Read the model definition and answer for the solid it produces. Units are mm, in the model's axes. Coordinates: 2 decimals unless noted, no trailing zeros. Write each loop counter-clockwise with the first axis right and the second up, starting at its lowest first coordinate (ties: lowest second). Pieces come first, ordered by that corner, then holes. Notation, with made-up numbers: (39.25, 61) -> (62.25, 61) arc R10 ccw to (62.25, 77) -> close; hole circle Ø10 at (62.25, 65.5). An arc over 180 degrees is marked (long way). Answer in a Markdown table with one row per item. Add a question column.
Item 1: Straight lines are drawn through the part: line 1 (Y direction, x = -1, z = -0.95); line 2 (X direction, y = 41, z = -3.4); line 3 (X direction, y = -46.5, z = -0.6). For each, find the intervals that lie inside material, in ascending order. Write a range as from..to.
Item 2: Section B-B on x = 25 is taken. Write down the section's boundary in (y, z), then the cut area to 3 significant figures.
Item 3: Section A-A on y = -127.5 is taken. Write down the section's boundary in (x, z), then the cut area to 3 significant figures.
Item 4: Given pin 1 Ø0.8 at (x, z) = (182, -3) entering from +Y; pin 2 Ø0.8 at (x, z) = (-61.5, -2) entering from -Y, each flat-ended and moving along its own axis, determine where each tip first touches the part or whether it passes through.
Item 5: Section C-C on z = -2.8 is taken. Count the separate pieces of the cut face and the enclosed holes in it, then the cut area to 3 significant figures.
```python
from build123d import *

# Parameters (mm, degrees)
BOSS_EXTRUDE1_DEPTH = 4.7625
SKETCH2_R           = 2.5
SKETCH2_W           = 35
SKETCH2_H           = 20
SKETCH2_W_2         = 1.5
SKETCH2_H_2         = 4
CUT_EXTRUDE1_DEPTH  = 10


with BuildPart() as part:
    # Sketch1 → Boss-Extrude1 (new body)
    with BuildSketch(Plane.XY):
        with BuildLine():
            Line((-66.942601108, 67.806403557), (-66.942601108, -242.193596443))
            ThreePointArc((-66.942601108, -242.193596443), (-64.599455358, -247.850450692), (-58.942601108, -250.193596443))
            Line((-58.942601108, -250.193596443), (179.057398892, -250.193596443))
            ThreePointArc((179.057398892, -250.193596443), (184.714253141, -247.850450692), (187.057398892, -242.193596443))
            Line((187.057398892, -242.193596443), (187.057398892, 67.806403557))
            ThreePointArc((187.057398892, 67.806403557), (184.714253141, 73.463257807), (179.057398892, 75.806403557))
            Line((179.057398892, 75.806403557), (-58.942601108, 75.806403557))
            ThreePointArc((-58.942601108, 75.806403557), (-64.599455358, 73.463257807), (-66.942601108, 67.806403557))
        make_face()
    extrude(amount=-BOSS_EXTRUDE1_DEPTH)

    # Sketch2 → Cut-Extrude1 (cut)
    with BuildSketch(Plane.XY):
        with Locations((179.057398892, 67.806403557)):
            Circle(SKETCH2_R)
        with Locations((-58.942601108, 67.806403557)):
            Circle(SKETCH2_R)
        with Locations((-58.942601108, -242.193596443)):
            Circle(SKETCH2_R)
        with Locations((179.057398892, -242.193596443)):
            Circle(SKETCH2_R)
        with BuildLine():
            Line((173.057398892, 25.806403557), (70.057398892, 25.806403557))
            ThreePointArc((70.057398892, 25.806403557), (66.521864986, 27.270869651), (65.057398892, 30.806403557))
            Line((65.057398892, 30.806403557), (65.057398892, 54.806403557))
            ThreePointArc((65.057398892, 54.806403557), (60.057398892, 59.806403557), (55.057398892, 54.806403557))
            Line((55.057398892, 54.806403557), (55.057398892, 30.806403557))
            ThreePointArc((55.057398892, 30.806403557), (53.592932798, 27.270869651), (50.057398892, 25.806403557))
            Line((50.057398892, 25.806403557), (-52.942601108, 25.806403557))
            Line((-52.942601108, 25.806403557), (-52.942601108, -200.193596443))
            Line((-52.942601108, -200.193596443), (173.057398892, -200.193596443))
            Line((173.057398892, -200.193596443), (173.057398892, 25.806403557))
        make_face()
        with Locations((-9.442601108, 49.806403557)):
            Rectangle(SKETCH2_W, SKETCH2_H)
        with Locations((129.557398892, 49.806403557)):
            Rectangle(SKETCH2_W, SKETCH2_H)
        with Locations((-61.692601108, 52.806403557)):
            Rectangle(SKETCH2_W_2, SKETCH2_H_2)
        with Locations((-52.192601108, 52.806403557)):
            Rectangle(SKETCH2_W_2, SKETCH2_H_2)
        with Locations((172.307398892, 52.806403557)):
            Rectangle(SKETCH2_W_2, SKETCH2_H_2)
        with Locations((181.807398892, 52.806403557)):
            Rectangle(SKETCH2_W_2, SKETCH2_H_2)
        with Locations((-9.442601108, -224.193596443)):
            Rectangle(SKETCH2_W, SKETCH2_H)
        with Locations((-61.692601108, -227.193596443)):
            Rectangle(SKETCH2_W_2, SKETCH2_H_2)
        with Locations((-52.192601108, -227.193596443)):
            Rectangle(SKETCH2_W_2, SKETCH2_H_2)
        with Locations((181.807398892, -227.193596443)):
            Rectangle(SKETCH2_W_2, SKETCH2_H_2)
        with Locations((172.307398892, -227.193596443)):
            Rectangle(SKETCH2_W_2, SKETCH2_H_2)
        with Locations((129.557398892, -224.193596443)):
            Rectangle(SKETCH2_W, SKETCH2_H)
    extrude(amount=-CUT_EXTRUDE1_DEPTH, mode=Mode.SUBTRACT)


solid = part.part
```
Results below:
| question | item | result |
|---|---|---|
| 1 | line 1 | y = -250.19..-234.19, -214.19..-200.19, 25.81..39.81, 59.81..75.81 |
| 1 | line 2 | x = -66.94..-26.94, 8.06..55.06, 65.06..112.06, 147.06..187.06 |
| 1 | line 3 | x = -66.94..-52.94, 173.06..187.06 |
| 2 | outline | (-250.19, -4.76) -> (-200.19, -4.76) -> (-200.19, 0) -> (-250.19, 0) -> close; (25.81, -4.76) -> (75.81, -4.76) -> (75.81, 0) -> (25.81, 0) -> close |
| 2 | area | 476 mm2 |
| 3 | outline | (-66.94, -4.76) -> (-52.94, -4.76) -> (-52.94, 0) -> (-66.94, 0) -> close; (173.06, -4.76) -> (187.06, -4.76) -> (187.06, 0) -> (173.06, 0) -> close |
| 3 | area | 133 mm2 |
| 4 | pin 1 | stops at y = 75.39 |
| 4 | pin 2 | stops at y = -249.9 |
| 5 | separate pieces | 1 |
| 5 | enclosed holes | 17 |
| 5 | area | 28,400 mm2 |
